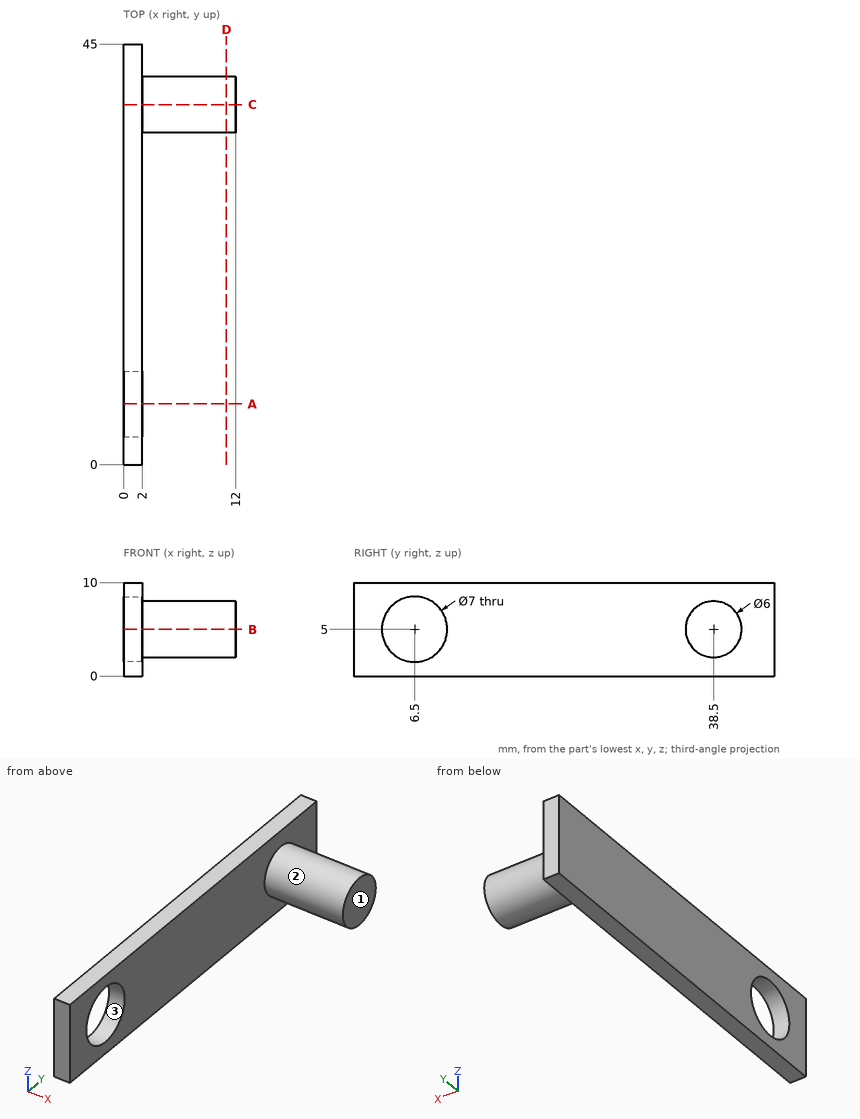
Geometry check sheet. Reference: drawing and pictorial views, mm from the part's lowest x, y, z. Give positions to 0.01 mm unless a question says otherwise; leave off trailing zeros. Order: outer loops, then holes, each group sorted by start corner. A loop starts at its lowest first (then second) coordinate and runs counter-clockwise, first axis right, second up. Notation, with made-up numbers: M 68.5,-6.75 L 107.5,-6.75 A30 ccw 107.5,23.25 Z; hole C 7.5,14 d10. An arc over 180 degrees is marked long. Answer as CSV lines item,"result". Start each with the question number.
Item 1: Cross-section at B-B on z = 5. Enter the section's corners in (x, y).
Item 2: Mould release check, pull along Y, two halves, no side actions. Record for the marked faces 1, 2 and 3: +Y half, -Y half, draft (parallel to the pull), parting line (faces both ways), or undercut.
Item 3: Gauge pin test, flat ends, axial feed: P1, Ø1.5, axis at x = 2, y = 4.5, coming from the -Z side; P2, Ø1, axis at y = 24.5, z = 4, coming from the +X side; P3, Ø2, axis at x = 5.5, z = 4, coming from the -Y side; P4, Ø5, axis at x = 5, z = 1.5, coming from the +Y side. Record the tip position at first contact, or that the pin passes through.
Item 4: Cross-section at A-A on y = 6.5. Enter the section's corners in (x, z).
Item 5: Thickness scan on line 1 (Y direction, x = 1.6, z = 5); line 2 (X direction, y = 29, z = 0.75); line 3 (Y direction, x = 1.5, z = 6). Record the ranges inside material, lowest first. Write a range as [from, to].
Item 6: Cross-section at C-C on y = 38.5. Enter the section's corners in (x, z), plus the area to 3 significant figures.
Item 7: Cross-section at D-D on x = 11. Enter the section's corners in (y, z).
Established:
1,outline,"M 0,0 L 2,0 L 2,3 L 0,3 Z; M 0,10 L 2,10 L 2,35.5 L 12,35.5 L 12,41.5 L 2,41.5 L 2,45 L 0,45 Z"
2,face 1,"draft"
2,face 2,"parting line"
2,face 3,"undercut"
3,P1,"stops at z = 0"
3,P2,"stops at x = 2"
3,P3,"stops at y = 35.5"
3,P4,"stops at y = 41.33"
4,outline,"M 0,0 L 2,0 L 2,1.5 L 0,1.5 Z; M 0,8.5 L 2,8.5 L 2,10 L 0,10 Z"
5,line 1,"y = [0, 3], [10, 45]"
5,line 2,"x = [0, 2]"
5,line 3,"y = [0, 3.15], [9.85, 45]"
6,outline,"M 0,0 L 2,0 L 2,2 L 12,2 L 12,8 L 2,8 L 2,10 L 0,10 Z"
6,area,"80.0 mm^2"
7,outline,"C 38.5,5 d6"
